from build123d import *

# Parameters (mm, degrees)
CROQUIS1_W                       = 52.1
CROQUIS1_H                       = 52.1
SALIENTE_EXTRUIR1_DEPTH          = 13
CROQUIS2_W                       = 42.1
CROQUIS2_H                       = 42.1
CORTAR_EXTRUIR1_DEPTH            = 12
SALIENTE_EXTRUIR2_DEPTH          = 3
TALADRO_DE_MARGEN_PARA_M31_D     = 3.4
TALADRO_START                    = 3
TALADRO_DE_MARGEN_PARA_M61_DEPTH = 10
REDONDEO1_R                      = 2
CROQUIS10_R                      = 5
CORTAR_EXTRUIR2_DEPTH            = 1
MATRIZC1_COUNT                   = 4
REDONDEO1_OF_MATRIZC1_R          = 2
CORTAR_EXTRUIR3_REACH            = 47.795
CROQUIS11_W                      = 32.1
CROQUIS11_H                      = 5
CORTAR_EXTRUIR4_REACH            = 68.284
CROQUIS12_R                      = 10
CROQUIS13_R                      = 1.5
SALIENTE_EXTRUIR3_DEPTH          = 1.5


# Read off the part's stored shape, not the designer's step: Taladro de margen para M61
with BuildPart() as part:
    # Croquis1 → Saliente-Extruir1 (new body)
    with BuildSketch(Plane.XY):
        Rectangle(CROQUIS1_W, CROQUIS1_H)
    extrude(amount=SALIENTE_EXTRUIR1_DEPTH)

    # Croquis2 → Cortar-Extruir1 (cut)
    with BuildSketch(Plane(origin=(0, 0, 0), x_dir=(-1, 0, 0), z_dir=(0, 0, -1))):
        Rectangle(CROQUIS2_W, CROQUIS2_H)
    extrude(amount=-CORTAR_EXTRUIR1_DEPTH, mode=Mode.SUBTRACT)

    # Croquis3 → Saliente-Extruir2 (add)
    with BuildSketch(Plane(origin=(0, 0, 0), x_dir=(-1, 0, 0), z_dir=(0, 0, -1))):
        Polygon((-31.05, 21.05), (-26.05, 16.05), (-26.05, 21.05), (-21.05, 21.05), (-21.05, 26.05), (-16.05, 26.05), (-21.05, 31.05), (-31.05, 31.05), align=None)
    saliente_extruir2 = extrude(amount=-SALIENTE_EXTRUIR2_DEPTH)

    # Taladro de margen para M31 (through all)
    with Locations(Plane(origin=(0, 0, 0), x_dir=(-1, 0, 0), z_dir=(0, 0, -1))):
        with Locations((-26.05, 26.05)):
            taladro_de_margen_para_m31 = Hole(TALADRO_DE_MARGEN_PARA_M31_D / 2)

    # Taladro de margen para M61 outline → Taladro de margen para M61 (cut)
    with BuildSketch(Plane.XY.offset(TALADRO_START)):
        with BuildLine():
            Line((24.35, 26.05), (22.75, 26.05))
            ThreePointArc((22.75, 26.05), (23.716547622, 23.716547622), (26.05, 22.75))
            Line((26.05, 22.75), (26.05, 24.35))
            ThreePointArc((26.05, 24.35), (24.847918472, 24.847918472), (24.35, 26.05))
        make_face()
    taladro_de_margen_para_m61 = extrude(amount=TALADRO_DE_MARGEN_PARA_M61_DEPTH, mode=Mode.SUBTRACT)

    # Redondeo1
    redondeo1_edges = [part.edges().sort_by_distance(p)[0] for p in [
        (31.05, 31.05, 1.5),
    ]]
    fillet(redondeo1_edges, radius=REDONDEO1_R)

    # Croquis10 → Cortar-Extruir2 (cut)
    with BuildSketch(Plane.XY.offset(13)):
        Circle(CROQUIS10_R)
    extrude(amount=-CORTAR_EXTRUIR2_DEPTH, mode=Mode.SUBTRACT)

    # MatrizC1: Saliente-Extruir2, Taladro de margen para M31, Taladro de margen para M61 ×4 about axis
    matrizc1_axis = Axis((0, 0, 0), (0, 0, 1))
    add([saliente_extruir2.rotate(matrizc1_axis, i * 360 / MATRIZC1_COUNT) for i in range(1, MATRIZC1_COUNT)])
    add([taladro_de_margen_para_m31.rotate(matrizc1_axis, i * 360 / MATRIZC1_COUNT) for i in range(1, MATRIZC1_COUNT)], mode=Mode.SUBTRACT)
    add([taladro_de_margen_para_m61.rotate(matrizc1_axis, i * 360 / MATRIZC1_COUNT) for i in range(1, MATRIZC1_COUNT)], mode=Mode.SUBTRACT)

    # Redondeo1 of MatrizC1
    redondeo1_of_matrizc1_edges = [part.edges().sort_by_distance(p)[0] for p in [
        (-31.05, 31.05, 1.5),
        (-31.05, -31.05, 1.5),
        (31.05, -31.05, 1.5),
    ]]
    fillet(redondeo1_of_matrizc1_edges, radius=REDONDEO1_OF_MATRIZC1_R)

    # Cortar-Extruir3: up to this face of the body (flat: up to its plane)
    cortar_extruir3_end = Plane(part.part.faces().sort_by_distance((20.45461609, 0, 12))[0])
    # Croquis11 → Cortar-Extruir3 (cut, up to the picked face)
    with BuildSketch(Plane(origin=(0, 0, 0), x_dir=(-1, 0, 0), z_dir=(0, 0, -1)), mode=Mode.PRIVATE) as cortar_extruir3_sk1:
        with Locations((0, 23.55)):
            Rectangle(CROQUIS11_W, CROQUIS11_H)
    cortar_extruir3_tool1 = split(extrude(cortar_extruir3_sk1.sketch, amount=-CORTAR_EXTRUIR3_REACH, mode=Mode.PRIVATE), bisect_by=cortar_extruir3_end, keep=Keep.BOTH, mode=Mode.PRIVATE)
    add(cortar_extruir3_tool1.solids().sort_by(Axis((0, 23.55, 0), (0, 0, 1)))[0], mode=Mode.SUBTRACT)

    # Cortar-Extruir4: up to this face of the body (flat: up to its plane)
    cortar_extruir4_end = Plane(part.part.faces().sort_by_distance((26.05, 0, 6.864592781))[0])
    # Croquis12 → Cortar-Extruir4 (cut, up to the picked face)
    with BuildSketch(Plane.ZY.offset(26.05), mode=Mode.PRIVATE) as cortar_extruir4_sk1:
        Circle(CROQUIS12_R)
    cortar_extruir4_tool1 = split(extrude(cortar_extruir4_sk1.sketch, amount=-CORTAR_EXTRUIR4_REACH, mode=Mode.PRIVATE), bisect_by=cortar_extruir4_end, keep=Keep.BOTH, mode=Mode.PRIVATE)
    add(cortar_extruir4_tool1.solids().sort_by(Axis((-26.05, 0, 0), (1, 0, 0)))[0], mode=Mode.SUBTRACT)

    # Croquis13 → Saliente-Extruir3 (add, symmetric)
    with BuildSketch(Plane(origin=(0, 0, 0), x_dir=(0, 0, -1), z_dir=(1, 0, 0))):
        Polygon((-13, 16.05), (-13, 31.05), (-18, 31.05), (-18, 16.05), (-13, 11.05), align=None)
        with Locations((-15.523423592, 28.55)):
            Circle(CROQUIS13_R, mode=Mode.SUBTRACT)
    saliente_extruir3 = extrude(amount=SALIENTE_EXTRUIR3_DEPTH, both=True)

    # Simetría1: Saliente-Extruir3 across plane
    add(saliente_extruir3.mirror(Plane.ZX))


solid = part.part
Work out the finished part from the listing and answer in its coordinate system (mm). A direction names the side the tool comes from. Coordinates: 2 decimals unless noted, no trailing zeros. Write each loop counter-clockwise with the first axis right and the second up, starting at its lowest first coordinate (ties: lowest second). Pieces come first, ordered by that corner, then holes. Notation, with made-up numbers: M 75,39 L 130,39 A20 ccw 130,47 Z; hole C 44.25,76 d11. An arc over 180 degrees is marked long. Use one line per item in the form item = value. Start each with the question number.
1. The part is cut by section A-A (y = 0). Give the vertices of the cut face in (x, z), plus the area to 3 significant figures.
2. The part is cut by section B-B (x = 2.5). Give the vertices of the cut face in (y, z).
3. Each of these flat-tipped pins is pushed along its axis until it touches: P1, Ø1, axis at y = -19, z = 9.5, coming from the -X side; P2, Ø21, axis at x = -8, y = 6, coming from the -Z side; P3, Ø1.5, axis at y = 19.5, z = 16.5, coming from the +X side. Where does it stop, or does it pass through?
4. The part is cut by section C-C (z = 7.75). Give the vertices of the cut face in (x, y), plus the area to 3 significant figures.
5. Straight lines are drawn through the part: probe 1 along X at (y, z) = (26.05, 1.45); probe 2 along X at (y, z) = (15, 2.5). For each, find the intervals that lie inside material, in ascending order. Write a range as from..to.
6. The mould has two halves that part along X. Classify faces 1 (the face through (23, 23, 0)), 2 (the face through (-26.05, 0, 11)), 3 (the face through (19, -29, 1)): released by +X, released by -X, zero draft, split by the parting line, or undercut.
7. The part is cut by section D-D (y = 19.5). Give the vertices of the cut face in (x, z).
8. A tool of negligible diameter and unlimited length cuts with its end or side. For faces 4 (the face through (26.05, 0, 11)), 5 (the face through (29, -27, 3)), 6 (the face through (-19, -29, 1)), 7 (the face through (-29, -27, 3)), 8 (the face through (-29, 27, 3)), from which of +Z, -Z, +X, -X, +Y, -Y can it reach the whole face along a straight path? Write none if from no direction.
Evaluation:
q1.outline = M -26.05,10 L -21.05,10 L -21.05,12 L -5,12 L -5,13 L -26.05,13 Z; M 5,12 L 21.05,12 L 21.05,10 L 26.05,10 L 26.05,13 L 5,13 Z
q1.area = 62.1 mm^2
q2.outline = M -26.05,0 L -21.05,0 L -21.05,12 L -4.33,12 L -4.33,13 L -26.05,13 Z; M 4.33,12 L 26.05,12 L 26.05,13 L 4.33,13 Z
q3.P1 = -26.05
q3.P2 = 12
q3.P3 = 1.5
q4.outline = M -26.05,-22.75 A3.3 cw -22.75,-26.05 L 22.75,-26.05 A3.3 cw 26.05,-22.75 L 26.05,-6.32 L 21.05,-6.32 L 21.05,-21.05 L -21.05,-21.05 L -21.05,-6.32 L -26.05,-6.32 Z; M -26.05,6.32 L -21.05,6.32 L -21.05,21.05 L -16.05,21.05 L -16.05,26.05 L -22.75,26.05 A3.3 cw -26.05,22.75 Z; M 16.05,21.05 L 21.05,21.05 L 21.05,6.32 L 26.05,6.32 L 26.05,22.75 A3.3 cw 22.75,26.05 L 16.05,26.05 Z
q4.area = 621 mm^2
q5.probe_1 = -31.05..-27.75, -24.35..-16.05, 16.05..24.35, 27.75..31.05
q5.probe_2 = -26.05..-21.05, 21.05..26.05
q6.face_1 = zero draft
q6.face_2 = released by -X
q6.face_3 = undercut
q7.outline = M -29.5,0 L -21.05,0 L -21.05,12 L 21.05,12 L 21.05,0 L 29.5,0 L 29.5,3 L 26.05,3 L 26.05,13 L 1.5,13 L 1.5,18 L -1.5,18 L -1.5,13 L -26.05,13 L -26.05,3 L -29.5,3 Z
q8.face_4 = +Z, +X
q8.face_5 = +Z, +X, -Y
q8.face_6 = +Z, -Z, -Y
q8.face_7 = +Z, -X, -Y
q8.face_8 = +Z, -X, +Y
